Here's how the part is built. I have some questions about the finished solid (model axes, mm). A direction names the side the tool comes from. Round coordinates to 2 decimals unless told otherwise and drop trailing zeros. One line per question, with ' | ' between items. Start each with the question number.
(1) Imagine slicing it at A-A (y = -0.55). Give the number of separate pieces and of enclosed holes in the cut face, plus the area to 3 significant figures.
(2) If I drill on L1, parallel to X at y = -0.05, z = 1.1; L2, parallel to X at y = -0.45, z = 1; L3, parallel to Y at x = 0.25, z = -1.8 (3 decimals), over which ranges is the centre line in solid material (lowest first)?
(3) Will these pins go through, and if not, where does the flat tip stop? pin 1 (1.5 mm diameter, centred on x = -2.5, z = -1, fed in from -Y) (3 decimals); pin 2 (2 mm diameter, centred on y = -0.5, z = 0.5, fed in from -X); pin 3 (1.2 mm diameter, centred on x = 3.5, y = -1.5, fed in from -Z).
(4) For faces 1 (the flat face through (0, -1.825, 0)), 2 (the flat face through (-2.715, 1.32, -0.031)), which set-ups out of +Z, -Z, +X, -X, +Y, -Y let a thin tool reach every point of the face, with its end or its side?
from build123d import *

# Parameters (mm, degrees)
SKETCH1_W                = 6.4
SKETCH1_H                = 4.58
EXTRUDE1_DEPTH           = 1.825
EXTRUDE1_TAPER           = 5
EXTRUDE1_OTHER_WAY_DEPTH = 1.825
EXTRUDE1_OTHER_WAY_TAPER = 5
CHAMFER1_SIZE            = 1
CHAMFER1_SIZE_2          = 0.748750861
EXTRUDE2_START           = 1.2
EXTRUDE2_DEPTH           = 0.3
FILLET1_R                = 0.1
FILLET2_R                = 0.35


with BuildPart() as part:
    # Sketch1 → Extrude1 (new body)
    with BuildSketch(Plane(origin=(0, 0, 0), x_dir=(1, 0, 0), z_dir=(0, 1, 0))):
        Rectangle(SKETCH1_W, SKETCH1_H)
    extrude(amount=EXTRUDE1_DEPTH, taper=EXTRUDE1_TAPER)

    # Sketch1 → Extrude1 other way (add)
    with BuildSketch(Plane(origin=(0, 0, 0), x_dir=(1, 0, 0), z_dir=(0, 1, 0))):
        Rectangle(SKETCH1_W, SKETCH1_H)
    extrude(amount=-EXTRUDE1_OTHER_WAY_DEPTH, taper=EXTRUDE1_OTHER_WAY_TAPER)

    # Chamfer1
    # the kernel refuses this chamfer: 1, 0.748750861 mm, written as the material it takes off along each edge
    with BuildSketch(Plane(origin=(-3.040333189, 1.825, -4.712885419), x_dir=(-0.10925940413866445, -0.9940132708406181, 0), z_dir=(0, 0, 1))) as chamfer1_piece_1:
        Polygon((CHAMFER1_SIZE * 0.999753334764, CHAMFER1_SIZE * 0.0222096741985), (-CHAMFER1_SIZE_2 * 0.109259404139, CHAMFER1_SIZE_2 * 0.994013270843), (0, 0), align=None)
    extrude(amount=9.425770839, mode=Mode.SUBTRACT)

    # Sketch2 → Extrude2 (add, symmetric)
    with BuildSketch(Plane.XY.offset(EXTRUDE2_START)):
        Polygon((-2.92973568, 0), (-3.42, 0), (-3.588415677, -1.925), (-4.288415677, -1.925), (-4.288415677, -1.675), (-3.817498471, -1.675), (-3.649082794, 0.25), (-2.92973568, 0.25), align=None)
        Polygon((2.92973568, 0.25), (2.92973568, 0), (3.42, 0), (3.588415677, -1.925), (4.288415677, -1.925), (4.288415677, -1.675), (3.817498471, -1.675), (3.649082794, 0.25), align=None)
    extrude2 = extrude(amount=EXTRUDE2_DEPTH, both=True)

    # Mirror1: Extrude2 across plane
    add(extrude2.mirror(Plane.XY))

    # Fillet1
    fillet1_edges = [part.edges().sort_by_distance(p)[0] for p in [
        (3.817498471, -1.675, -1.2),
        (3.42, 0, -1.2),
        (-3.817498471, -1.675, 1.2),
        (-3.42, 0, 1.2),
        (3.42, 0, 1.2),
        (3.817498471, -1.675, 1.2),
        (-3.42, 0, -1.2),
        (-3.817498471, -1.675, -1.2),
    ]]
    fillet(fillet1_edges, radius=FILLET1_R)

    # Fillet2
    fillet2_edges = [part.edges().sort_by_distance(p)[0] for p in [
        (3.649082794, 0.25, -1.2),
        (3.588415677, -1.925, -1.2),
        (-3.649082794, 0.25, 1.2),
        (-3.588415677, -1.925, 1.2),
        (3.649082794, 0.25, 1.2),
        (3.588415677, -1.925, 1.2),
        (-3.649082794, 0.25, -1.2),
        (-3.588415677, -1.925, -1.2),
    ]]
    fillet(fillet2_edges, radius=FILLET2_R)


solid = part.part
Check sheet entries:
1) separate pieces: 5 | enclosed holes: 0 | area: 28.9 mm^2
2) L1: -3.67 to -3.41, -3.2 to 3.2, 3.41 to 3.67 | L2: -3.71 to -3.46, -3.16 to 3.16, 3.46 to 3.71 | L3: -1.825 to 1.825
3) pin 1: y = -1.825 | pin 2: x = -3.79 | pin 3: z = -2.2
4) face 1: +Z, -Z, -Y | face 2: +Z, -Z, -X, +Y
